Can you work these out from the model? Positions are in its coordinate system, mm. A direction names the side the tool comes from. Give positions to 0.01 mm unless a question says otherwise; leave off trailing zeros. Order: outer loops, then holes, each group sorted by start corner. A loop starts at its lowest first (then second) coordinate and runs counter-clockwise, first axis right, second up. Notation, with made-up numbers: (37.5, 87) - (74.5, 87) arc R13 cw to (74.5, 92) - close; hole circle Ø5 at (63.25, 47.25). An arc over 180 degrees is marked (long way). Return JSON: item names as keys, results as strings.
```python
from build123d import *

# Parameters (mm, degrees)
RESSALTO_EXTRUS_O2_DEPTH = 12.8


with BuildPart() as part:
    # Esboço1 → Ressalto-extrusão2 (new body)
    with BuildSketch(Plane(origin=(0, 0, 0), x_dir=(1, 0, 0), z_dir=(0, 1, 0))):
        with BuildLine():
            Line((-27.75, 25.45), (27.75, 25.45))
            Line((27.75, 25.45), (31.75, 21.45))
            Line((31.75, 21.45), (31.75, 16.9))
            Line((31.75, 16.9), (16.264213562, 1.414213562))
            ThreePointArc((16.264213562, 1.414213562), (15.678427125, 0), (16.264213562, -1.414213562))
            Line((16.264213562, -1.414213562), (31.75, -16.9))
            Line((31.75, -16.9), (31.75, -21.45))
            Line((31.75, -21.45), (27.75, -25.45))
            Line((27.75, -25.45), (-27.75, -25.45))
            Line((-27.75, -25.45), (-31.75, -21.45))
            Line((-31.75, -21.45), (-31.75, 21.45))
            Line((-31.75, 21.45), (-27.75, 25.45))
        make_face()
        with BuildLine():
            Line((-25.3, 7.65), (-6.6, 7.65))
            ThreePointArc((-6.6, 7.65), (-3.8, 4.85), (-6.6, 2.05))
            Line((-6.6, 2.05), (-25.3, 2.05))
            ThreePointArc((-25.3, 2.05), (-28.1, 4.85), (-25.3, 7.65))
        make_face(mode=Mode.SUBTRACT)
    extrude(amount=RESSALTO_EXTRUS_O2_DEPTH)


solid = part.part
```
1. Thinking about a two-plate mould opening in Z: for faces 4 (the face through (-29.8, 6.3, -23.4)), 5 (the face through (-28.1, 6.3, -4.8)), 6 (the face through (31.75, 6, 19)), which applies, +Z half, -Z half, draft (parallel to the pull), parting line (faces both ways), or undercut?
Checks:
{"face 4": "-Z half", "face 5": "undercut", "face 6": "draft"}
2. If I drill on L1, parallel to Z at x = -7, y = 1.75; L2, parallel to Z at x = 24, y = 4.25; L3, parallel to X at y = 1.75, z = -13, over which ranges is the centre line in solid material (lowest first)? Write a range as [from, to].
Checks:
{"L1": "[-25.45, -7.65], [-2.05, 25.45]", "L2": "[-25.45, -9.15], [9.15, 25.45]", "L3": "[-31.75, 27.85]"}
3. Suppose I cut it at C-C (y = 4.25). List the corners of the cut face in (x, z) for me, plus the area to 3 significant figures.
Checks:
{"outline": "(-31.75, -21.45) - (-27.75, -25.45) - (27.75, -25.45) - (31.75, -21.45) - (31.75, -16.9) - (16.26, -1.41) arc R2 cw to (16.26, 1.41) - (31.75, 16.9) - (31.75, 21.45) - (27.75, 25.45) - (-27.75, 25.45) - (-31.75, 21.45) - close; hole (-25.3, -7.65) - (-6.6, -7.65) arc R2.8 ccw to (-6.6, -2.05) - (-25.3, -2.05) arc R2.8 ccw to start", "area": "2,790 mm^2"}
4. Suppose I cut it at B-B (x = -12). List the corners of the cut face in (y, z) for me.
Checks:
{"outline": "(0, -25.45) - (12.8, -25.45) - (12.8, -7.65) - (0, -7.65) - close; (0, -2.05) - (12.8, -2.05) - (12.8, 25.45) - (0, 25.45) - close"}
5. Suppose I cut it at D-D (z = 10). List the corners of the cut face in (x, y) for me, plus the area to 3 significant figures.
Checks:
{"outline": "(-31.75, 0) - (24.85, 0) - (24.85, 12.8) - (-31.75, 12.8) - close", "area": "724 mm^2"}
6. Suppose I cut it at A-A (z = -4.85). List the corners of the cut face in (x, y) for me, plus the area to 3 significant figures.
Checks:
{"outline": "(-31.75, 0) - (-28.1, 0) - (-28.1, 12.8) - (-31.75, 12.8) - close; (-3.8, 0) - (19.7, 0) - (19.7, 12.8) - (-3.8, 12.8) - close", "area": "348 mm^2"}
7. On a 3-axis mill with a long thin cutter (end or side, diameter ignored), from which of +Z, -Z, +X, -X, +Y, -Y can I reach the whole of each face in a straight line? I mean faces 1 (the face through (29.8, 6.3, 23.4)), 2 (the face through (24.12, 6.31, -9.27)), 3 (the face through (-16, 6, -7.65)). Say none if no direction works.
Checks:
{"face 1": "+Z, +X, +Y, -Y", "face 2": "+X, +Y, -Y", "face 3": "+Y, -Y"}
8. For pin 1 Ø3 at (y, z) = (5.5, 2) entering from +X, with a flat end and sliding along its axis, tell me the tip position at first contact or that it passes through.
Checks:
{"pin 1": "x = 18.35"}
